Can you work these out from the model? Positions are in its coordinate system, mm. A direction names the side the tool comes from. Give positions to 0.01 mm unless a question says otherwise; leave off trailing zeros. Write each loop counter-clockwise with the first axis right and the second up, starting at its lowest first coordinate (ties: lowest second). Pieces come first, ordered by that corner, then holes.
from build123d import *

# Parameters (mm, degrees)
BOSS_EXTRUDE1_DEPTH = 5


with BuildPart() as part:
    # Sketch1 → Boss-Extrude1 (new body)
    with BuildSketch(Plane.XY):
        with BuildLine():
            Line((5.550510257, 0.824633862), (7.550510257, 0.824633862))
            ThreePointArc((7.550510257, 0.824633862), (6.500182239, 3.288917717), (7.5, 5.774123605))
            Line((7.5, 5.774123605), (7.5, 8.824633862))
            Line((7.5, 8.824633862), (12.5, 8.824633862))
            Line((12.5, 8.824633862), (12.5, 5.774123605))
            ThreePointArc((12.5, 5.774123605), (13.499817761, 3.288917717), (12.449489743, 0.824633862))
            Line((12.449489743, 0.824633862), (14.449489743, 0.824633862))
            Line((14.449489743, 0.824633862), (20, 4))
            Line((20, 4), (20, 8.824633862))
            Line((20, 8.824633862), (17.5, 8.824633862))
            Line((17.5, 8.824633862), (17.5, 13.824633862))
            Line((17.5, 13.824633862), (10, 13.824633862))
            Line((10, 13.824633862), (2.5, 13.824633862))
            Line((2.5, 13.824633862), (2.5, 8.824633862))
            Line((2.5, 8.824633862), (0, 8.824633862))
            Line((0, 8.824633862), (0, 4))
            Line((0, 4), (5.550510257, 0.824633862))
        make_face()
    extrude(amount=BOSS_EXTRUDE1_DEPTH)


solid = part.part
(1) Imagine slicing it at A-A, the plane y = 8. Write out the boundary of the cut face in (x, z).
Returned:
outline: (0, 0) - (7.5, 0) - (7.5, 5) - (0, 5) - close; (12.5, 0) - (20, 0) - (20, 5) - (12.5, 5) - close
(2) Imagine slicing it at D-D, the plane x = 11.25. Write out the boundary of the cut face in (y, z), plus the area to 3 significant figures.
Returned:
outline: (8.82, 0) - (13.82, 0) - (13.82, 5) - (8.82, 5) - close
area: 25.0 mm2
(3) Imagine slicing it at B-B, the plane z = 4. Write out the boundary of the cut face in (x, y).
Returned:
outline: (0, 4) - (5.55, 0.82) - (7.55, 0.82) arc R3.5 cw to (7.5, 5.77) - (7.5, 8.82) - (12.5, 8.82) - (12.5, 5.77) arc R3.5 cw to (12.45, 0.82) - (14.45, 0.82) - (20, 4) - (20, 8.82) - (17.5, 8.82) - (17.5, 13.82) - (2.5, 13.82) - (2.5, 8.82) - (0, 8.82) - close
(4) Will this pin go through, and if not, where does the flat tip stop? P1, Ø2, axis at y = 10.5, z = 2.5, coming from the -X side.
Returned:
P1: stops at x = 2.5
(5) If I drill on L1, parallel to X at y = 7, z = 3.5; L2, parallel to X at y = 9.5, z = 2.8; L3, parallel to X at y = 5.5, z = 2.9, over which ranges is the centre line in solid material (lowest first)?
Returned:
L1: x = 0 to 7.5, 12.5 to 20
L2: x = 2.5 to 17.5
L3: x = 0 to 7.26, 12.74 to 20
(6) Imagine slicing it at C-C, the plane y = 1.5. Write out the boundary of the cut face in (x, z).
Returned:
outline: (4.37, 0) - (7.01, 0) - (7.01, 5) - (4.37, 5) - close; (12.99, 0) - (15.63, 0) - (15.63, 5) - (12.99, 5) - close
(7) For faces 4 (the face through (19, 8.825, 2)), 5 (the face through (10, 13.825, 2)), 6 (the face through (1, 8.825, 2)), 7 (the face through (12.5, 7, 2)), which set-ups out of +Z, -Z, +X, -X, +Y, -Y let a thin tool reach every point of the face, with its end or its side?
Returned:
face 4: +Z, -Z, +X, +Y
face 5: +Z, -Z, +X, -X, +Y
face 6: +Z, -Z, -X, +Y
face 7: +Z, -Z
(8) If we mould it in two halves opening along X, with no side actions, what happens to faces 1 (the face through (10, 9, 0)), 2 (the face through (2.5, 11, 2)), 3 (the face through (6.5, 3.3, 2.5))? For each: +X half, -X half, draft (parallel to the pull), parting line (faces both ways), or undercut.
Returned:
face 1: draft
face 2: -X half
face 3: undercut
